Autodesk Inventor part; units mm, degrees
ref_plane "YZ Plane" through (0, 0, 0) normal (1, 0, 0) x (0, 1, 0)
ref_plane "XZ Plane" through (0, 0, 0) normal (0, 1, 0) x (-1, 0, 0)
ref_plane "XY Plane" through (0, 0, 0) normal (0, 0, 1) x (1, 0, 0)
sketch "Sketch1" plane through (0, 0, 0) normal (0, 0, 1) x (1, 0, 0)
  circle A0 centre (0, 0) radius 4.7625
  circle A1 centre (0, 0) radius 11.1125
  dimension "d0" = 9.525
  dimension "d1" = 22.225
extrude "Extrusion1" add sketch "Sketch1" along normal blind 1.27
sketch "Sketch2" plane through (0, 0, 1.27) normal (0, 0, 1) x (1, 0, 0)
  circle A0 centre (0, 8.3312) radius 1.651
  circle A1 centre (-7.215, -4.1656) radius 1.651
  circle A2 centre (7.215, -4.1656) radius 1.651
  point P0 (0, 0)
  dimension "d4" = 3.302
  dimension "d7" = 360
  dimension "d9" = 8.3312
extrude "Extrusion2" cut sketch "Sketch2" against normal blind 1.27
properties part number "CompressionWasherPlastic" material "ABS Plastic"
Could you check a few things on this model? Use its own coordinates, in mm. Round coordinates to 2 decimals unless told otherwise and drop trailing zeros. Loops run counter-clockwise (first coordinate to the right, second up) from the corner with the lowest first, then second, coordinate; pieces in that order, holes last. Notation, with made-up numbers: M -11.75,-12.75 L 31.25,-12.75 A34 cw 31.25,17.25 Z; hole C -36.5,83 d9. An arc over 180 degrees is marked long. Put each result on its own line as item: value.
Q1. Imagine slicing it at A-A (x = 0). Write out the boundary of the cut face in (y, z).
Check result:
outline: M -11.11,0 L -4.76,0 L -4.76,1.27 L -11.11,1.27 Z; M 4.76,0 L 6.68,0 L 6.68,1.27 L 4.76,1.27 Z; M 9.98,0 L 11.11,0 L 11.11,1.27 L 9.98,1.27 Z
Q2. I need wall thicknesses on probe 1 along Y at (x, z) = (0, 0.4); probe 2 along Y at (x, z) = (1.5, 0.7); probe 3 along Y at (x, z) = (8, 0.3). Which ranges of each line are inside material? Lowest first, please.
Check result:
probe 1: -11.11 to -4.76, 4.76 to 6.68, 9.98 to 11.11
probe 2: -11.01 to -4.52, 4.52 to 7.64, 9.02 to 11.01
probe 3: -7.71 to -5.62, -2.71 to 7.71
Q3. Imagine slicing it at C-C (y = -3.25). Write out the boundary of the cut face in (x, z).
Check result:
outline: M -10.63,0 L -8.59,0 L -8.59,1.27 L -10.63,1.27 Z; M -5.84,0 L -3.48,0 L -3.48,1.27 L -5.84,1.27 Z; M 3.48,0 L 5.84,0 L 5.84,1.27 L 3.48,1.27 Z; M 8.59,0 L 10.63,0 L 10.63,1.27 L 8.59,1.27 Z
Q4. Imagine slicing it at D-D (z = 0.2). Write out the boundary of the cut face in (x, y) (1 decimal), then the cut area to 3 significant figures.
Check result:
outline: C 0,0 d22.2; hole C -7.2,-4.2 d3.3; hole C 0,0 d9.5; hole C 0,8.3 d3.3; hole C 7.2,-4.2 d3.3
area: 291 mm2
Q5. Thinking about a two-plate mould opening in Y: for faces 1 (the face through (-3.78, 2.9, 0.63)), 2 (the face through (10.6, -3.34, 0.63)), 3 (the face through (-8.43, -3.05, 0.64)), 4 (the face through (5, 0, 0)), which applies, released by +Y, released by -Y, zero draft, split by the parting line, or undercut?
Check result:
face 1: undercut
face 2: split by the parting line
face 3: undercut
face 4: zero draft
Q6. Imagine slicing it at B-B (y = 0). Write out the boundary of the cut face in (x, z).
Check result:
outline: M -11.11,0 L -4.76,0 L -4.76,1.27 L -11.11,1.27 Z; M 4.76,0 L 11.11,0 L 11.11,1.27 L 4.76,1.27 Z
